Verification items for the finished model (mm, model axes). A direction names the side the tool comes from. Give positions to 0.01 mm unless a question says otherwise; leave off trailing zeros. Order: outer loops, then holes, each group sorted by start corner. A loop starts at its lowest first (then second) coordinate and runs counter-clockwise, first axis right, second up. Notation, with made-up numbers: (-27, 27) -> (-1, 27) arc R35 ccw to (-1, 62) -> close; hole circle Ø10 at (49.25, 9). An arc over 180 degrees is marked (long way). Return JSON: item names as keys, results as strings. Group by question number.
(1) Cross-section at D-D on y = 27.5. Enter the section's corners in (x, z).
(2) Cross-section at A-A on x = -33. Enter the section's corners in (y, z).
(3) Tool access check on faces 1 (the face through (-58.549, -13, 68)), 2 (the face through (61.451, -13, 68)), 3 (the face through (1, -42, 15)), 4 (the face through (2, -36.935, 68)). Record the directions out of +Z, -Z, +X, -X, +Y, -Y that give a thin tool (end or side, any length) a straight path to the whole face; none if there is none.
(4) Depth check by flat-ended pin: pin 1 Ø10 at (y, z) = (7.5, 89.5) entering from -X; pin 2 Ø6 at (y, z) = (11.5, 100.5) entering from +X; pin 3 Ø3.5 at (x, z) = (47.21, 69.18) entering from +Y. Enter the tip coordinate at first touch or a pass-through.
(5) Cross-section at B-B on y = 13. Enter the section's corners in (x, z), then the cut area to 3 significant figures.
(6) Cross-section at C-C on z = 53.5. Enter the section's corners in (x, y).
(7) Thickness scan on line 1 along Z through (x, y) = (0, -40); line 2 along Z through (x, y) = (-48.5, 8); line 3 along X through (y, z) = (17.5, 82). Record the ranges inside material, lowest first.
(8) Release check for a two-part mould opening along Z. For faces 5 (the face through (1, -14, 125)), 6 (the face through (-64.035, -2, 5)), 7 (the face through (0, -1, 0)), 8 (the face through (-53.575, -9, 67)) record: pulls with the +Z half, pulls with the -Z half, needs draft (parallel to the pull), parting line crosses it, or undercut.
from build123d import *

# Parameters (mm, degrees)
F0_W     = 130
F0_H     = 75
F1_DEPTH = 10
F2_W     = 120
F2_H     = 57.4860367924
F3_DEPTH = 5
F5_DEPTH = 120
F7_D     = 2.794
F8_W     = 109.1061495245
F8_H     = 106.3687205315
F8_R     = 1.397
F9_DEPTH = 55


with BuildPart() as f1:
    # F0 (on Top) → F1 (new body)
    with BuildSketch(Plane.XY):
        with Locations((0.9653219581, -1.9211560488)):
            Rectangle(F0_W, F0_H)
    extrude(amount=F1_DEPTH)

    # F2 (on face) → F3 (join)
    with BuildSketch(Plane.XY.offset(10)):
        with Locations((1.4508789778, -10.6781376526)):
            Rectangle(F2_W, F2_H)
    extrude(amount=F3_DEPTH)

    # F4 (on face) → F5 (join)
    with BuildSketch(Plane(origin=(-58.5491210222, 0, 0), x_dir=(0, -1, 0), z_dir=(-1, 0, 0))):
        Polygon((-18.0648807436, 125), (-18.0648807436, 15), (39.4211560488, 15), (45.2204495668, 15), (45.2204495668, 125), align=None)
    extrude(amount=-F5_DEPTH)

    # F7 (through all)
    with Locations(Plane.XZ.offset(45.2204495668)):
        with Locations((0, 116.3231828261), (-47.0786592322, 69.1776266678), (0, 22.0320705095), (47.2125481423, 69.1776266678), (0.066944455, 69.1776266678)):
            Hole(F7_D / 2)

    # F8 (on face) → F9 (cut)
    with BuildSketch(Plane(origin=(0, 18.0648807436, 0), x_dir=(-1, 0, 0), z_dir=(0, 1, 0))):
        with Locations((-0.9776521474, 67.4301683903)):
            Rectangle(F8_W, F8_H)
        with Locations((0, 22.0320705095)):
            Circle(F8_R, mode=Mode.SUBTRACT)
        with Locations((-47.2125481423, 69.1776266678)):
            Circle(F8_R, mode=Mode.SUBTRACT)
        with Locations((-0.066944455, 69.1776266678)):
            Circle(F8_R, mode=Mode.SUBTRACT)
        with Locations((47.0786592322, 69.1776266678)):
            Circle(F8_R, mode=Mode.SUBTRACT)
        with Locations((0, 116.3231828261)):
            Circle(F8_R, mode=Mode.SUBTRACT)
    extrude(amount=-F9_DEPTH, mode=Mode.SUBTRACT)


solid = f1.part
Verdict:
{
 "1": {"outline": "(-64.03, 0) -> (65.97, 0) -> (65.97, 10) -> (-64.03, 10) -> close"},
 "2": {"outline": "(-45.22, 15) -> (-39.42, 15) -> (-39.42, 0) -> (35.58, 0) -> (35.58, 10) -> (18.06, 10) -> (18.06, 14.25) -> (-36.94, 14.25) -> (-36.94, 120.61) -> (18.06, 120.61) -> (18.06, 125) -> (-45.22, 125) -> close"},
 "3": {"face 1": "+Z, -X, +Y, -Y", "face 2": "+Z, +X, +Y, -Y", "face 3": "-Z, +X, -X, -Y", "face 4": "+Y"},
 "4": {"pin 1": "x = -58.55", "pin 2": "x = 61.45", "pin 3": "y = -36.94"},
 "5": {"outline": "(-64.03, 0) -> (65.97, 0) -> (65.97, 10) -> (61.45, 10) -> (61.45, 125) -> (-58.55, 125) -> (-58.55, 10) -> (-64.03, 10) -> close; hole (-53.58, 14.25) -> (55.53, 14.25) -> (55.53, 120.61) -> (-53.58, 120.61) -> close", "area": "3,490 mm²"},
 "6": {"outline": "(-58.55, -45.22) -> (61.45, -45.22) -> (61.45, 18.06) -> (55.53, 18.06) -> (55.53, -36.94) -> (-53.58, -36.94) -> (-53.58, 18.06) -> (-58.55, 18.06) -> close"},
 "7": {"line 1": "15 to 20.64, 23.43 to 67.78, 70.57 to 114.93, 117.72 to 125", "line 2": "0 to 14.25, 120.61 to 125", "line 3": "-58.55 to -53.58, 55.53 to 61.45"},
 "8": {"face 5": "pulls with the +Z half", "face 6": "needs draft", "face 7": "pulls with the -Z half", "face 8": "undercut"}
}
